Autodesk Inventor part; units mm, degrees
ref_plane "YZ Plane" through (0, 0, 0) normal (1, 0, 0) x (0, 1, 0)
ref_plane "XZ Plane" through (0, 0, 0) normal (0, 1, 0) x (-1, 0, 0)
ref_plane "XY Plane" through (0, 0, 0) normal (0, 0, 1) x (1, 0, 0)
sketch "Boceto6" plane through (0, 0, 0) normal (1, 0, 0) x (0, 1, 0)
  line L0 (0, 0) -> (180, 0)
  line L1 (180, 0) -> (180, -10)
  line L2 (180, -10) -> (0, -10)
  line L3 (0, -10) -> (0, 0)
  dimension "d12" = 180
  dimension "d13" = 10
extrude "Extrusión3" add sketch "Boceto6" along normal mid plane 45.3
sketch "Boceto7" plane through (22.65, 0, 0) normal (1, 0, 0) x (0, 0, -1)
  line L0 (10, 0) -> (10, 180)
  line L1 (10, 180) -> (0, 180)
  line L2 (10, 180) -> (0, 180)
  line L3 (0, 180) -> (-14.8492, 194.8492)
  line L4 (10, 180) -> (-9.8492, 199.8492)
  line L5 (10, 180) -> (38.0711, 180) construction
  line L6 (-9.8492, 199.8492) -> (-14.8492, 194.8492)
  point P0 (0, 0)
  dimension "d16" = 21
  dimension "d17" = 135
  dimension "d18" = 135
extrude "Extrusión4" add sketch "Boceto7" against normal blind 45.3
sketch "Boceto8" plane through (22.65, 180, -10) normal (0, 0.7071, -0.7071) x (-1, 0, 0)
  circle A0 centre (10.275, 15) radius 8
  circle A1 centre (34.725, 15) radius 8
  line L0 (0, 0) -> (0, 28.0711)
  line L1 (45.3, 0) -> (0, 0)
  point P0 (22.65, -120.2082)
  dimension "d21" = 16
  dimension "d22" = 16
  dimension "d23" = 24.45
  dimension "d24" = 10.275
  dimension "d25" = 15
  dimension "d26" = 15
extrude "Extrusión5" cut sketch "Boceto8" against normal blind 8.25
sketch "Boceto11" plane through (22.65, 180, -10) normal (0, 0.7071, -0.7071) x (-1, 0, 0)
  circle A0 centre (1.95, 23.0711) radius 1.5
  line L0 (0, 0) -> (0, 28.0711)
  line L1 (0, 28.0711) -> (45.3, 28.0711)
  circle A1 centre (43.35, 7) radius 1.5
  line L2 (45.3, 28.0711) -> (45.3, 0)
  line L3 (45.3, 0) -> (0, 0)
  point P0 (22.65, -120.2082)
  point P1 (45.5, 0)
  dimension "d29" = 3
  dimension "d30" = 1.95
  dimension "d31" = 5
  dimension "d32" = 3
  dimension "d33" = 1.95
  dimension "d34" = 7
extrude "Extrusión6" cut sketch "Boceto11" against normal blind 12.5 contours A0 | A1
sketch "Boceto12" plane through (22.65, 0, -10) normal (0, 0, -1) x (-1, 0, 0)
  line L0 (0, 0) -> (0, 180)
  line L1 (0, 7) -> (45.3, 7)
  line L2 (45.3, 7) -> (45.3, 0)
  line L3 (45.3, 0) -> (0, 0)
  line L4 (0, 0) -> (0, 7)
  line L5 (0, 0) -> (45.3, 0)
  point P0 (22.65, 0)
  point P1 (22.65, 0)
  dimension "d37" = 7
  dimension "d38" = 0
extrude "Extrusión7" add sketch "Boceto12" along normal blind 20.5
sketch "Boceto13" plane through (-22.65, 0, 0) normal (0, 0, 1) x (1, 0, 0)
  line L0 (0, 0) -> (0, 180)
  line L1 (0, 7) -> (45.3, 7)
  line L2 (45.3, 7) -> (45.3, 0)
  line L3 (45.3, 0) -> (0, 0)
  line L4 (0, 0) -> (0, 7)
  line L5 (0, 0) -> (45.3, 0)
  point P0 (22.65, 0)
  dimension "d41" = 7
  dimension "d42" = 0
extrude "Extrusión8" add sketch "Boceto13" along normal blind 20.5
sketch "Boceto15" plane through (-22.65, 0, -30.5) normal (0, -1, 0) x (1, 0, 0)
  circle A0 centre (7.95, 45.3492) radius 1.5
  line L0 (45.3, 45.3492) -> (0, 45.3492)
  circle A1 centre (37.95, 45.3492) radius 1.5
  line L1 (0, 51) -> (45.3, 51)
  circle A2 centre (7.95, 5.6508) radius 1.5
  circle A3 centre (37.95, 5.6508) radius 1.5
  line L2 (45.3, 0) -> (0, 0)
  line L3 (45.3, 0) -> (45.3, 51)
  point P0 (22.65, 30.5)
  dimension "d45" = 3
  dimension "d46" = 3
  dimension "d47" = 5.6508
  dimension "d48" = 3
  dimension "d49" = 3
  dimension "d50" = 5.6508
  dimension "d51" = 5.6508
  dimension "d52" = 30
  dimension "d53" = 30
  dimension "d54" = -7.35
  dimension "d55" = -7.35
extrude "Extrusión9" cut sketch "Boceto15" against normal blind 20.5
equation "\"d50\" = d47"
equation "\"d51\" = d47"
equation "\"d55\" = d54"
properties part number "Soporte_Ultrasonido"
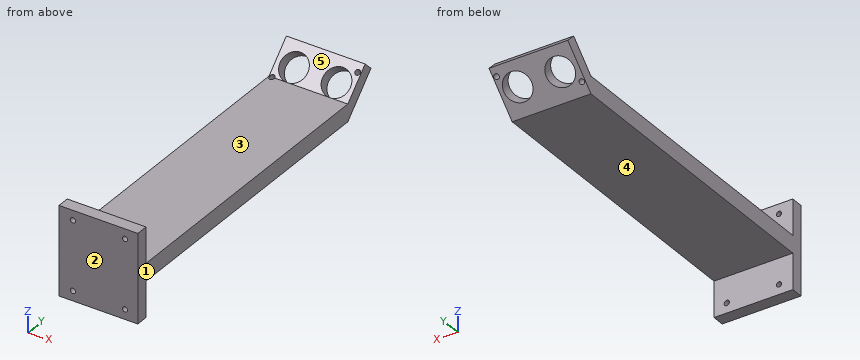
Check sheet for the modelled part. Datum: model origin and axes. Units: mm. Face numbers are marked on the shaded views. A direction names the side the tool comes from. Give positions to 0.01 mm unless a question says otherwise; leave off trailing zeros. Write each loop counter-clockwise with the first axis right and the second up, starting at its lowest first coordinate (ties: lowest second). Pieces come first, ordered by that corner, then holes. Notation, with made-up numbers: M 50.5,-35 L 78.5,-35 A29 cw 78.5,0 Z; hole C -20,59 d2. An arc over 180 degrees is marked long. Use one line per item in the form item = value.
(1) Depth check by flat-ended pin: P1, Ø10, axis at y = 70, z = 4, coming from the +X side; P2, Ø10, axis at x = 5.5, z = -22.5, coming from the +Y side; P3, Ø1.8, axis at x = -14.7, z = -24.85, coming from the -Y side; P4, Ø12, axis at x = -13.5, y = 72, coming from the -Z side. Enter the tip coordinate at first touch or a pass-through.
Answer block:
P1 = 22.65
P2 = 7
P3 = through
P4 = -10
(2) Tool access check on the marked faces 4 and 5. Record the directions out of +Z, -Z, +X, -X, +Y, -Y that give a thin tool (end or side, any length) a straight path to the whole face; none if there is none.
Answer block:
face_4 = -Z, +X, -X, +Y
face_5 = +Z, +X, -X
(3) Material ranges on line 1 along Z through (x, y) = (15, 3); line 2 along Z through (x, y) = (15.3, 3.75); line 3 along Y through (x, z) = (20, 7.5), recorded low to high.
Answer block:
line_1 = -30.5 to -26.32, -23.38 to 13.38, 16.32 to 20.5
line_2 = -30.5 to -26.35, -23.35 to 13.35, 16.35 to 20.5
line_3 = 0 to 7, 187.5 to 193.25, 197 to 197.5
(4) Section check A-A on x = 7.5. Record the boundary of the cut face in (y, z), plus the area to 3 significant figures.
Answer block:
outline = M 0,-30.5 L 7,-30.5 L 7,-10 L 180,-10 L 186.12,-3.88 L 181.12,1.12 L 180,0 L 7,0 L 7,20.5 L 0,20.5 Z; M 190.09,10.09 L 195.09,5.09 L 199.85,9.85 L 194.85,14.85 Z
area = 2,170 mm2
(5) Draft check along Y on the marked faces 1, 2 and 3. Enter one of: pulls with the +Y half, pulls with the -Y half, needs draft (parallel to the pull), parting line crosses it, or undercut.
Answer block:
face_1 = needs draft
face_2 = pulls with the -Y half
face_3 = undercut
(6) Section check B-B on z = -20. Record the boundary of the cut face in (x, y), plus the area to 3 significant figures.
Answer block:
outline = M -22.65,0 L 22.65,0 L 22.65,7 L -22.65,7 Z
area = 317 mm2
(7) Section check C-C on y = 39.5. Record the boundary of the cut face in (x, z), plus the area to 3 significant figures.
Answer block:
outline = M -22.65,-10 L 22.65,-10 L 22.65,0 L -22.65,0 Z
area = 453 mm2
